```python
from build123d import *

# Parameters (mm, degrees)
CUT_EXTRUDE_1_DEPTH = 3.5


with BuildPart() as part:
    # 草图1 → 旋转1 (revolve)
    with BuildSketch(Plane.XY, mode=Mode.PRIVATE) as revolve_1_sk:
        with BuildLine():
            Line((0, 39), (-4.5, 39))
            ThreePointArc((-4.5, 39), (-4.782842712, 38.882842712), (-4.9, 38.6))
            Line((-4.9, 38.6), (-4.9, 35.4))
            ThreePointArc((-4.9, 35.4), (-4.782842712, 35.117157288), (-4.5, 35))
            Line((-4.5, 35), (-2.5, 35))
            Line((-2.5, 35), (-2.5, 33))
            Line((-2.5, 33), (-3, 33))
            Line((-3, 33), (-3, 10))
            Line((-3, 10), (-2, 10))
            Line((-2, 10), (-2, 8))
            Line((-2, 8), (-2.5, 8))
            Line((-2.5, 8), (-2.5, 0))
            Line((-2.5, 0), (0, 0))
            Line((0, 0), (0, 39))
        make_face()
    revolve(revolve_1_sk.sketch.rotate(Axis((0, 0, 0), (0, 1, 0)), 270), axis=Axis((0, 0, 0), (0, 1, 0)))

    # 草图2 → 切除-拉伸1 (cut)
    with BuildSketch(Plane(origin=(0, 39, 0), x_dir=(1, 0, 0), z_dir=(0, 1, 0))):
        Polygon((0.866025404, 1.5), (-0.866025404, 1.5), (-1.732050808, 0), (-0.866025404, -1.5), (0.866025404, -1.5), (1.732050808, 0), align=None)
    extrude(amount=-CUT_EXTRUDE_1_DEPTH, mode=Mode.SUBTRACT)


solid = part.part
```
Verification items for the finished model (mm, model axes). A direction names the side the tool comes from. Coordinates: 2 decimals unless noted, no trailing zeros. Loops run counter-clockwise (first coordinate to the right, second up) from the corner with the lowest first, then second, coordinate; pieces in that order, holes last. Notation, with made-up numbers: (-34, -22.75) -> (11, -22.75) arc R23 ccw to (11, 12.25) -> close; hole circle Ø3 at (23.25, 1). An arc over 180 degrees is marked (long way). Answer in a Markdown table with one row per item.
1) Draft check along Z on faces 1 (the face through (2.44, 3.94, 0.54)), 2 (the face through (-2, 33, -2)), 3 (the face through (0, 35.5, 0)), 4 (the face through (1.293, 37.274, 0.76)). Enter one of: released by +Z, released by -Z, zero draft, split by the parting line, or undercut.
The answers:
| item | result |
|---|---|
| face 1 | split by the parting line |
| face 2 | zero draft |
| face 3 | undercut |
| face 4 | undercut |
2) Section check B-B (y = 22). Record the cut outline in (x, z), and give its area (3 significant figures).
The answers:
| item | result |
|---|---|
| outline | circle Ø6 at (0, 0) |
| area | 28.3 mm2 |
3) Depth check by flat-ended pin: P1, Ø1.5, axis at x = -0.5, y = 12.5, coming from the -Z side; P2, Ø1.5, axis at x = 1, y = 4, coming from the -Z side; P3, Ø3, axis at x = -3.5, y = 30.5, coming from the -Z side. Enter the tip coordinate at first touch or a pass-through.
The answers:
| item | result |
|---|---|
| P1 | stops at z = -3 |
| P2 | stops at z = -2.49 |
| P3 | stops at z = -2.24 |
4) Access from +Z, -Z, +X, -X, +Y, -Y to the whole of each face (thin tool, end or side, straight path). Record for faces 5 (the face through (-1.305, 37.274, 0.74)), 6 (the face through (2, 9, 0)), 7 (the face through (-0.9, 21.34, -2.86)).
The answers:
| item | result |
|---|---|
| face 5 | +Y |
| face 6 | none |
| face 7 | -Y |
5) Scan lines: line 1 along Y through (x, z) = (-1.25, -2.5); line 2 along Y through (x, z) = (2, 0.5); line 3 along Y through (x, z) = (3.75, 1.5). Record each from-to range of solid material in increasing order. Write a range as from..to.
The answers:
| item | result |
|---|---|
| line 1 | y = 10..33, 35..39 |
| line 2 | y = 0..8, 10..39 |
| line 3 | y = 35..39 |
6) Section check A-A (x = 0). Record the cut outline in (y, z).
The answers:
| item | result |
|---|---|
| outline | (0, -2.5) -> (8, -2.5) -> (8, -2) -> (10, -2) -> (10, -3) -> (33, -3) -> (33, -2.5) -> (35, -2.5) -> (35, -4.5) arc R0.4 ccw to (35.4, -4.9) -> (38.6, -4.9) arc R0.4 ccw to (39, -4.5) -> (39, -1.5) -> (35.5, -1.5) -> (35.5, 1.5) -> (39, 1.5) -> (39, 4.5) arc R0.4 ccw to (38.6, 4.9) -> (35.4, 4.9) arc R0.4 ccw to (35, 4.5) -> (35, 2.5) -> (33, 2.5) -> (33, 3) -> (10, 3) -> (10, 2) -> (8, 2) -> (8, 2.5) -> (0, 2.5) -> close |
